Input: part model. Units: mm. Frame: model coordinates. A direction names the side the tool comes from. Give positions to 0.01 mm unless a question says otherwise; leave off trailing zeros. Loops run counter-clockwise (first coordinate to the right, second up) from the corner with the lowest first, then second, coordinate; pieces in that order, holes last. Notation, with made-up numbers: (74, 16) -> (124, 16) arc R26 ccw to (124, 55) -> close; hole circle Ø10 at (85.5, -7). An arc over 180 degrees is marked (long way). Answer as a JSON object with one key per item and string values. Group by question number.
```python
from build123d import *

# Parameters (mm, degrees)
SKETCH_W        = 9.6
SKETCH_H        = 9.6
PAD_DEPTH       = 10
SKETCH002_W     = 12
SKETCH002_H     = 12
PAD001_DEPTH    = 1
SKETCH003_W     = 3
SKETCH003_H     = 6
POCKET_DEPTH    = 9
SKETCH004_W     = 3
SKETCH004_H     = 6
POCKET001_DEPTH = 9
POCKET002_DEPTH = 11.001
POCKET003_DEPTH = 11.001
POCKET004_DEPTH = 11.001
POCKET005_DEPTH = 11.001
FILLET_R        = 1


with BuildPart() as part:
    # Sketch → Pad (new body)
    with BuildSketch(Plane.XY):
        Rectangle(SKETCH_W, SKETCH_H)
    extrude(amount=PAD_DEPTH)

    # Sketch002 → Pad001 (join)
    with BuildSketch(Plane(origin=(0, 0, 0), x_dir=(1, 0, 0), z_dir=(0, 0, -1))):
        Rectangle(SKETCH002_W, SKETCH002_H)
    extrude(amount=PAD001_DEPTH)

    # Sketch003 → Pocket (cut)
    with BuildSketch(Plane(origin=(0, 0, -2), x_dir=(1, 0, 0), z_dir=(0, 0, -1))):
        with Locations((-2.5, 0)):
            Rectangle(SKETCH003_W, SKETCH003_H)
    extrude(amount=-POCKET_DEPTH, mode=Mode.SUBTRACT)

    # Sketch004 → Pocket001 (cut)
    with BuildSketch(Plane(origin=(0, 0, -2), x_dir=(1, 0, 0), z_dir=(0, 0, -1))):
        with Locations((2.5, 0)):
            Rectangle(SKETCH004_W, SKETCH004_H)
    extrude(amount=-POCKET001_DEPTH, mode=Mode.SUBTRACT)

    # Sketch001 → Pocket002 (cut, through all)
    with BuildSketch(Plane.XY.offset(10)):
        Polygon((3.32, -0.5), (3.32, -2.95), (0.5, -2.95), (0.5, -2.45), (2.76, -2.45), (2.76, -0.5), align=None)
    extrude(amount=-POCKET002_DEPTH, mode=Mode.SUBTRACT)

    # Sketch005 → Pocket003 (cut, through all)
    with BuildSketch(Plane.XY.offset(10)):
        Polygon((-3.32, -0.5), (-3.32, -2.95), (-0.5, -2.95), (-0.5, -2.45), (-2.76, -2.45), (-2.76, -0.5), align=None)
    extrude(amount=-POCKET003_DEPTH, mode=Mode.SUBTRACT)

    # Sketch007 → Pocket004 (cut, through all)
    with BuildSketch(Plane.XY.offset(10)):
        Polygon((-2.76, 0.5), (-3.32, 0.5), (-3.32, 2.95), (-0.5, 2.95), (-0.5, 2.39), (-2.76, 2.39), align=None)
    extrude(amount=-POCKET004_DEPTH, mode=Mode.SUBTRACT)

    # Sketch006 → Pocket005 (cut, through all)
    with BuildSketch(Plane.XY.offset(10)):
        Polygon((0.5, 2.95), (3.32, 2.95), (3.32, 0.5), (2.76, 0.5), (2.76, 2.45), (0.5, 2.45), align=None)
    extrude(amount=-POCKET005_DEPTH, mode=Mode.SUBTRACT)

    # Fillet
    fillet_edges = [part.edges().sort_by_distance(p)[0] for p in [
        (0, 4.8, 10),
        (4.8, 0, 10),
        (0, -4.8, 10),
        (4.8, -4.8, 5),
        (4.8, 4.8, 5),
        (-4.8, 0, 10),
        (-4.8, -4.8, 5),
        (-4.8, 4.8, 5),
    ]]
    fillet(fillet_edges, radius=FILLET_R)


solid = part.part
```
Q1. Section C-C on z = 3.5. State how many separate pieces and enclosed holes the cut face has, then the cut area to 3 significant figures.
Q2. Ray query, probe 1 along X at (y, z) = (1.25, 8); probe 2 along Y at (x, z) = (1.25, 8.25); probe 3 along X at (y, z) = (-0.5, 5.5). Return the intervals inside material, ascending.
Q3. Pull-direction query (Y, two-part tool) for faces 5 (the face through (4.499, 4.515, 4.563)), 6 (the face through (-3, -3, 3)), 7 (the face through (0, 0, -1)), 8 (the face through (2, 3, 3)); classes: +Y half, -Y half, draft (parallel to the pull), parting line (faces both ways), or undercut.
Q4. Set-up query: faces 1 (the face through (-3, 3, 3)), 2 (the face through (4.8, 0, 4)), 3 (the face through (-6, 0.1, -0.5)), 4 (the face through (3.32, 2, 9)). Return all of +Z, -Z, +X, -X, +Y, -Y with unobstructed straight access to the full face (end or side cutting, diameter ignored); none if empty.
Q5. Section B-B on x = 1.75. Return the cut outline in (y, z), then the cut area to 3 significant figures.
Q6. Section D-D on x = -0.25. Return the cut outline in (y, z).
Q7. Section A-A on y = -1. Return the cut outline in (x, z).
Q8. Pin query (flat end, axial travel): pin 1 Ø1 at (x, z) = (-2.5, 6) entering from +Y; pin 2 Ø1.6 at (y, z) = (-2, 8.5) entering from +X; pin 3 Ø1.8 at (y, z) = (-0.5, 5) entering from -X. Return the tip coordinate at first contact, or that it passes through.
Numbers:
{
 "1": {"separate pieces": "1", "enclosed holes": "2", "area": "54.3 mm²"},
 "2": {"probe 1": "x = -4.8 to -3.32, -2.76 to 2.76, 3.32 to 4.8", "probe 2": "y = -4.8 to -2.95, -2.45 to 2.45, 2.95 to 4.8", "probe 3": "x = -4.8 to -4, -1 to 1, 4 to 4.8"},
 "3": {"face 5": "+Y half", "face 6": "undercut", "face 7": "draft", "face 8": "undercut"},
 "4": {"face 1": "-Z", "face 2": "+Z, +X, +Y, -Y", "face 3": "+Z, -Z, -X, +Y, -Y", "face 4": "+Z, -Z"},
 "5": {"outline": "(-6, -1) -> (-3, -1) -> (-3, 7) -> (-2.95, 7) -> (-2.95, 10) -> (-3.8, 10) arc R1 ccw to (-4.8, 9) -> (-4.8, 0) -> (-6, 0) -> close; (-2.45, 7) -> (2.45, 7) -> (2.45, 10) -> (-2.45, 10) -> close; (2.95, 7) -> (3, 7) -> (3, -1) -> (6, -1) -> (6, 0) -> (4.8, 0) -> (4.8, 9) arc R1 ccw to (3.8, 10) -> (2.95, 10) -> close", "area": "56.6 mm²"},
 "6": {"outline": "(-6, -1) -> (6, -1) -> (6, 0) -> (4.8, 0) -> (4.8, 9) arc R1 ccw to (3.8, 10) -> (-3.8, 10) arc R1 ccw to (-4.8, 9) -> (-4.8, 0) -> (-6, 0) -> close"},
 "7": {"outline": "(-6, -1) -> (-4, -1) -> (-4, 7) -> (-3.32, 7) -> (-3.32, 10) -> (-3.8, 10) arc R1 ccw to (-4.8, 9) -> (-4.8, 0) -> (-6, 0) -> close; (-2.76, 7) -> (-1, 7) -> (-1, -1) -> (1, -1) -> (1, 7) -> (2.76, 7) -> (2.76, 10) -> (-2.76, 10) -> close; (3.32, 7) -> (4, 7) -> (4, -1) -> (6, -1) -> (6, 0) -> (4.8, 0) -> (4.8, 9) arc R1 ccw to (3.8, 10) -> (3.32, 10) -> close"},
 "8": {"pin 1": "stops at y = 4.8", "pin 2": "stops at x = 4.8", "pin 3": "stops at x = -4.8"}
}
